Can you work these out from the model? Positions are in its coordinate system, mm. Face numbers are marked on the shaded views. A direction names the side the tool comes from. Round coordinates to 2 decimals unless told otherwise and drop trailing zeros. Order: outer loops, then holes, each group sorted by start corner. A loop starts at its lowest first (then second) coordinate and runs counter-clockwise, first axis right, second up.
from build123d import *

# Parameters (mm, degrees)
SKETCH_1_R               = 13.945
EXTRUDE_1_DEPTH          = 5.5
SKETCH_2_R               = 16
EXTRUDE_2_DEPTH          = 2
EXTRUDE_START            = 2
SKETCH_3_R               = 16
EXTRUDE_3_DEPTH          = 2
CUT_EXTRUDE_1_DEPTH      = 28.147743921
CUT_EXTRUDE_1_DEPTH_BACK = 28.147743921
SKETCH_4_R               = 2.5


with BuildPart() as part:
    # 草图1 → 凸台-拉伸1 (new, symmetric)
    with BuildSketch(Plane.XY):
        Circle(SKETCH_1_R)
    extrude(amount=EXTRUDE_1_DEPTH, both=True)

    # 草图2 → 凸台-拉伸2 (add)
    with BuildSketch(Plane.XY.offset(5.5)):
        Circle(SKETCH_2_R)
    extrude(amount=EXTRUDE_2_DEPTH)

    # 草图3 → 凸台-拉伸3 (add)
    with BuildSketch(Plane(origin=(0, 0, -5.5), x_dir=(-1, 0, 0), z_dir=(0, 0, -1)).offset(EXTRUDE_START)):
        with Locations(Location((0, 0, 0), (0, 0, 180))):
            Circle(SKETCH_3_R)
    extrude(amount=-EXTRUDE_3_DEPTH)

    # 草图4 → 切除-拉伸1 (cut, two sides: drawn at the far end of the back side and taken through both)
    with BuildSketch(Plane(origin=(0, 0, -7.5), x_dir=(-1, 0, 0), z_dir=(0, 0, -1)).offset(-CUT_EXTRUDE_1_DEPTH_BACK)):
        Circle(SKETCH_4_R)
    extrude(amount=CUT_EXTRUDE_1_DEPTH + CUT_EXTRUDE_1_DEPTH_BACK, mode=Mode.SUBTRACT)


solid = part.part
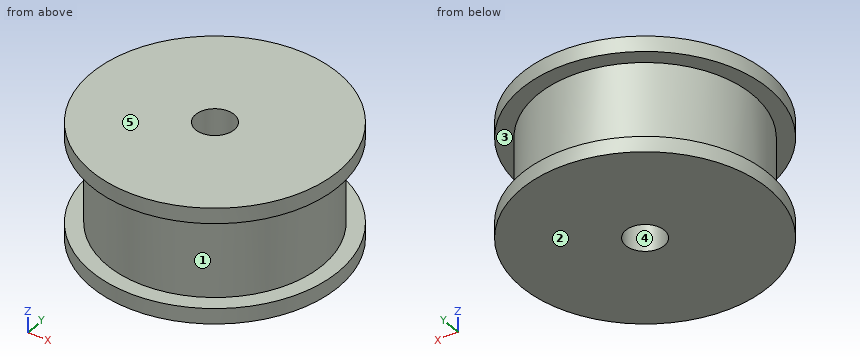
(1) I'm going to push flat-ended pins straight in: pin 1 Ø4 at (y, z) = (5.5, -1) entering from +X; pin 2 Ø3 at (y, z) = (8.5, 1.5) entering from +X; pin 3 Ø6 at (x, z) = (6, -6) entering from -Y. Where does each tip first touch, or does it pass through?
(2) I want a section at A-A, the plane x = 0. List the corners of the cut face in (y, z) for me (3 decimals), plus the area to 3 significant figures.
(3) If we mould it in two halves opening along Z, with no side actions, what happens to the marked faces 3, 4 and 5? For each: pulls with the +Z half, pulls with the -Z half, needs draft (parallel to the pull), parting line crosses it, or undercut.
(4) I want a section at D-D, the plane x = 13. List the corners of the cut face in (y, z) for me, plus the area to 3 significant figures.
(5) I want a section at C-C, the plane z = -1.75. List the corners of the cut face in (x, y) for me (3 decimals), plus the area to 3 significant figures.
(6) On a 3-axis mill with a long thin cutter (end or side, diameter ignored), from which of +Z, -Z, +X, -X, +Y, -Y can I reach the whole of each face in a straight line? I mean the marked faces 1 and 2. Say none if no direction works.
(7) Please list where these lines run through material, in increasing order: probe 1 along Y at (x, z) = (0, 0) (3 decimals); probe 2 along Z at (x, y) = (13, -6.5); probe 3 along X at (y, z) = (-1, 0).
Ans:
1. pin 1: stops at x = 13.5
1. pin 2: stops at x = 12.06
1. pin 3: stops at y = -15.72
2. outline: (-16, -7.5) - (-2.5, -7.5) - (-2.5, 7.5) - (-16, 7.5) - (-16, 5.5) - (-13.945, 5.5) - (-13.945, -5.5) - (-16, -5.5) - close; (2.5, -7.5) - (16, -7.5) - (16, -5.5) - (13.945, -5.5) - (13.945, 5.5) - (16, 5.5) - (16, 7.5) - (2.5, 7.5) - close
2. area: 360 mm2
3. face 3: undercut
3. face 4: needs draft
3. face 5: pulls with the +Z half
4. outline: (-9.33, -7.5) - (9.33, -7.5) - (9.33, -5.5) - (5.05, -5.5) - (5.05, 5.5) - (9.33, 5.5) - (9.33, 7.5) - (-9.33, 7.5) - (-9.33, 5.5) - (-5.05, 5.5) - (-5.05, -5.5) - (-9.33, -5.5) - close
4. area: 186 mm2
5. outline: circle Ø27.89 at (0, 0); hole circle Ø5 at (0, 0)
5. area: 591 mm2
6. face 1: none
6. face 2: -Z, +X, -X, +Y, -Y
7. probe 1: y = -13.945 to -2.5, 2.5 to 13.945
7. probe 2: z = -7.5 to -5.5, 5.5 to 7.5
7. probe 3: x = -13.91 to -2.29, 2.29 to 13.91
